Design review of the part built by this model. Coordinates are the model's own, in mm. Face numbers are marked on the shaded views. A direction names the side the tool comes from. Give positions to 0.01 mm unless a question says otherwise; leave off trailing zeros. Order: outer loops, then holes, each group sorted by start corner. A loop starts at its lowest first (then second) coordinate and runs counter-clockwise, first axis right, second up. Notation, with made-up numbers: M 4,-24.5 L 10,-24.5 A15 cw 10,4.5 Z; hole C 80,-22 d5. An arc over 180 degrees is marked long. Answer as a JSON object with one key per item and string values.
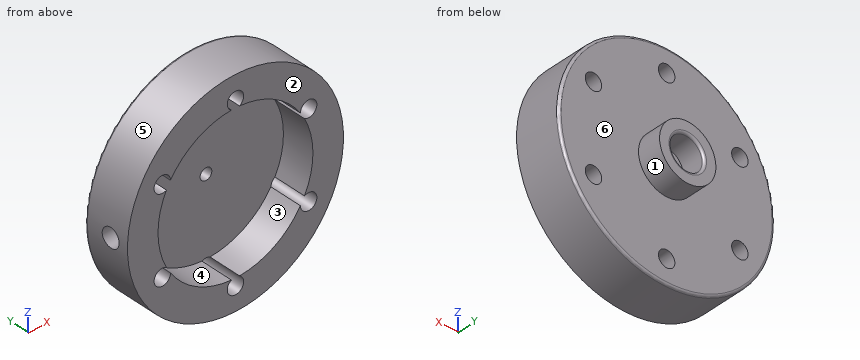
from build123d import *

# Parameters (mm, degrees)
SKETCH1_R           = 46
SKETCH1_R_2         = 3.5
BOSS_EXTRUDE1_DEPTH = 20
FILLET1_R           = 1
SKETCH2_R           = 12
BOSS_EXTRUDE2_DEPTH = 10
SKETCH3_R           = 33
CUT_EXTRUDE1_DEPTH  = 14
SKETCH4_R           = 2.5
CUT_EXTRUDE2_DEPTH  = 6
SKETCH5_R           = 7
CUT_EXTRUDE3_DEPTH  = 10
FILLET2_R           = 1
SKETCH6_R           = 4
CUT_EXTRUDE4_DEPTH  = 54


with BuildPart() as part:
    # Sketch1 → Boss-Extrude1 (new body)
    with BuildSketch(Plane(origin=(0, 0, 0), x_dir=(1, 0, 0), z_dir=(0, 1, 0))):
        with Locations(Location((0, 0, 0), (0, 0, 270))):
            Circle(SKETCH1_R)
        with Locations(Location((0, 36, 0), (0, 0, 270))):
            Circle(SKETCH1_R_2, mode=Mode.SUBTRACT)
        with Locations(Location((31.176914536, 18, 0), (0, 0, 270))):
            Circle(SKETCH1_R_2, mode=Mode.SUBTRACT)
        with Locations(Location((31.176914536, -18, 0), (0, 0, 270))):
            Circle(SKETCH1_R_2, mode=Mode.SUBTRACT)
        with Locations(Location((0, -36, 0), (0, 0, 270))):
            Circle(SKETCH1_R_2, mode=Mode.SUBTRACT)
        with Locations(Location((-31.176914536, -18, 0), (0, 0, 270))):
            Circle(SKETCH1_R_2, mode=Mode.SUBTRACT)
        with Locations(Location((-31.176914536, 18, 0), (0, 0, 270))):
            Circle(SKETCH1_R_2, mode=Mode.SUBTRACT)
    extrude(amount=BOSS_EXTRUDE1_DEPTH)

    # Fillet1
    fillet1_edges = [part.edges().sort_by_distance(p)[0] for p in [
        (0, 20, -46),
    ]]
    fillet(fillet1_edges, radius=FILLET1_R)

    # Sketch2 → Boss-Extrude2 (add)
    with BuildSketch(Plane(origin=(0, 20, 0), x_dir=(1, 0, 0), z_dir=(0, 1, 0))):
        with Locations(Location((0, 0, 0), (0, 0, 270))):
            Circle(SKETCH2_R)
    extrude(amount=BOSS_EXTRUDE2_DEPTH)

    # Sketch3 → Cut-Extrude1 (cut)
    with BuildSketch(Plane.XZ):
        Circle(SKETCH3_R)
    extrude(amount=-CUT_EXTRUDE1_DEPTH, mode=Mode.SUBTRACT)

    # Sketch4 → Cut-Extrude2 (cut)
    with BuildSketch(Plane.XZ.offset(-14)):
        with Locations(Location((0, 0, 0), (0, 0, 270))):
            Circle(SKETCH4_R)
    extrude(amount=-CUT_EXTRUDE2_DEPTH, mode=Mode.SUBTRACT)

    # Sketch5 → Cut-Extrude3 (cut)
    with BuildSketch(Plane(origin=(0, 30, 0), x_dir=(1, 0, 0), z_dir=(0, 1, 0))):
        with Locations(Location((0, 0, 0), (0, 0, 270))):
            Circle(SKETCH5_R)
    extrude(amount=-CUT_EXTRUDE3_DEPTH, mode=Mode.SUBTRACT)

    # Fillet2
    fillet2_edges = [part.edges().sort_by_distance(p)[0] for p in [
        (0, 30, -7),
    ]]
    fillet(fillet2_edges, radius=FILLET2_R)

    # Sketch6 → Cut-Extrude4 (cut)
    with BuildSketch(Plane(origin=(0, 0, 0), x_dir=(0, 0, -1), z_dir=(1, 0, 0))):
        with Locations((0, 8)):
            Circle(SKETCH6_R)
    extrude(amount=-CUT_EXTRUDE4_DEPTH, mode=Mode.SUBTRACT)


solid = part.part
(1) We need section B-B (z = 0). Write out the cut boundary in (x, y), plus the area to 3 significant figures.
Checked values:
{"outline": "M -46,0 L -33,0 L -33,4 L -46,4 Z; M -46,12 L -33,12 L -33,14 L -2.5,14 L -2.5,20 L -7,20 L -7,29 A1 ccw -8,30 L -12,30 L -12,20 L -45,20 A1 ccw -46,19 Z; M 2.5,14 L 33,14 L 33,0 L 46,0 L 46,19 A1 ccw 45,20 L 12,20 L 12,30 L 8,30 A1 ccw 7,29 L 7,20 L 2.5,20 Z", "area": "881 mm^2"}
(2) To check wall thickness, follow L1, parallel to X at y = 11, z = 20.5; L2, parallel to Z at x = -30, y = 7; L3, parallel to Y at x = 6.5, z = -5. State the ranges of each line that lie inside material, in increasing order. Write a range as from..to.
Checked values:
{"L1": "x = -41.18..-33.63, -28.73..-25.86, 25.86..28.73, 33.63..41.18", "L2": "z = -34.87..-21.3, -14.7..-13.75, 13.75..14.7, 21.3..34.87", "L3": "y = 14..30"}
(3) We need section C-C (y = 25). Write out the cut boundary in (x, z).
Checked values:
{"outline": "C 0,0 d24; hole C 0,0 d14"}
(4) Tool access review of the marked faces 1, 2 and 3: name each direction out of +Z, -Z, +X, -X, +Y, -Y from which nothing blocks a thin tool from reaching the whole face with its end or side.
Checked values:
{"face 1": "+Y", "face 2": "+Z, -Z, +X, -X, -Y", "face 3": "-Y"}
(5) Draft analysis for pull direction Z (two halves, no side actions). For the marked faces 4, 5 and 6, state which applies: +Z half, -Z half, draft (parallel to the pull), parting line (faces both ways), or undercut.
Checked values:
{"face 4": "undercut", "face 5": "parting line", "face 6": "draft"}
(6) We need section D-D (y = 8). Write out the cut boundary in (x, z).
Checked values:
{"outline": "M -45.83,-4 A46 ccw long -45.83,4 L -32.76,4 A33 cw -29.4,14.98 A3.5 cw long -27.68,17.97 A33 cw -1.73,32.95 A3.5 cw long 1.73,32.95 A33 cw 27.68,17.97 A3.5 cw long 29.4,14.98 A33 cw 29.4,-14.98 A3.5 cw long 27.68,-17.97 A33 cw 1.73,-32.95 A3.5 cw long -1.73,-32.95 A33 cw -27.68,-17.97 A3.5 cw long -29.4,-14.98 A33 cw -32.76,-4 Z"}
(7) Insertion check: pin 1 (1.5 mm diameter, centred on x = 27, z = 16, fed in from -Y); pin 2 (1.5 mm diameter, centred on x = 26.5, y = 15.5, fed in from -Z); pin 3 (1 mm diameter, centred on y = 21.5, z = -11, fed in from +X); pin 4 (4.5 mm diameter, centred on x = 0, z = 0, fed in from -Y) (3 decimals). Each pin has a flat end and moves straight along its axis. Give the tip position at first contact, or say it passes through.
Checked values:
{"pin 1": "stops at y = 14", "pin 2": "stops at z = -38.12", "pin 3": "stops at x = 5.81", "pin 4": "passes through"}
(8) We need section A-A (x = 0). Write out the cut boundary in (y, z), plus the area to 3 significant figures.
Checked values:
{"outline": "M 0,-46 L 19,-46 A1 ccw 20,-45 L 20,-39.5 L 0,-39.5 Z; M 0,39.5 L 20,39.5 L 20,45 A1 ccw 19,46 L 0,46 Z; M 14,-32.5 L 20,-32.5 L 20,-12 L 30,-12 L 30,-8 A1 ccw 29,-7 L 20,-7 L 20,-2.5 L 14,-2.5 Z; M 14,2.5 L 20,2.5 L 20,7 L 29,7 A1 ccw 30,8 L 30,12 L 20,12 L 20,32.5 L 14,32.5 Z", "area": "719 mm^2"}
